Geometry: final body of the model. Coordinates: model frame, mm. A direction names the side the tool comes from. Give positions to 0.01 mm unless a question says otherwise; leave off trailing zeros. Write each loop counter-clockwise with the first axis right and the second up, starting at its lowest first coordinate (ties: lowest second). Pieces come first, ordered by that corner, then holes. Notation, with made-up numbers: (59, -2.5) - (63, -2.5) arc R16 ccw to (63, 12.5) - close; hole circle Ø4 at (-38, 41). An arc over 180 degrees is marked (long way). Use CSV: the item, a comma, the result in double quotes. Start each with the question number.
(1) Line query: probe 1 along X at (y, z) = (244, 98.5); probe 2 along Y at (x, z) = (22.5, 80.5); probe 3 along X at (y, z) = (36, 24.5). Output: solid intervals per line, ascending. Write a range as [from, to].
(2) Section C-C on x = 12. Output: boundary loops of the cut face in (y, z) (3 decimals).
(3) First-contact query: pin 1 Ø1.5 at (x, z) = (184, 43) entering from +Y; pin 2 Ø4 at (y, z) = (277.477, 41.275) entering from +X; pin 3 Ø1.5 at (y, z) = (193.5, 71.5) entering from +X. Flat tips, straight axial feed; report the tip coordinate or a pass-through.
(4) Section B-B on y = 248. Output: boundary loops of the cut face in (x, z) (3 decimals), and give its area (3 significant figures).
(5) Section A-A on z = 89. Output: boundary loops of the cut face in (x, y) (3 decimals).
(6) Reachability of faces 1 (the flat face through (-55.496, 208, 58)), 2 (the flat face through (141.09, -19.38, 57.92)) from +Z, -Z, +X, -X, +Y, -Y: full face, straight path, thin tool, end or side. Return the list, or none.
Autodesk Inventor part; units mm, degrees
ref_plane "YZ Plane" through (0, 0, 0) normal (1, 0, 0) x (0, 1, 0)
ref_plane "XZ Plane" through (0, 0, 0) normal (0, 1, 0) x (-1, 0, 0)
ref_plane "XY Plane" through (0, 0, 0) normal (0, 0, 1) x (1, 0, 0)
sketch "Sketch1" plane through (0, 0, 0) normal (0, 0, 1) x (1, 0, 0)
  line L0 (-58.6709, 290.177) -> (-55.4959, 290.177)
  line L1 (-58.6709, 290.177) -> (-58.6709, 129.0683)
  arc A0 (-58.6709, 129.0683) -> (52.835, -3.8192) centre (76.2666, 129.0683) ccw
  line L2 (52.835, -3.8192) -> (231.8416, -35.3829)
  line L3 (231.8416, -32.1589) -> (231.8416, -35.3829)
  line L4 (231.8416, -32.1589) -> (53.3863, -0.6924)
  arc A1 (-55.4959, 129.0683) -> (53.3863, -0.6924) centre (76.2666, 129.0683) ccw
  line L5 (-55.4959, 129.0683) -> (-55.4959, 290.177)
  point P0 (0, 0)
extrude "Extrusion1" add sketch "Sketch1" along normal blind 117.475
hole "Hole1" at (-55.4959, 277.477, 109.5375) direction (-1, 0, 0) diameter 6.731 depth 25.4 tip angle 118
pattern_linear "Rectangular Pattern1" count 2 spacing 133.35 along (0, -1, 0) of "Hole1"
pattern_linear "Rectangular Pattern2" count 2 spacing 68.2625 along (0, 0, -1) of "Hole1"
hole "Hole2" at (219.3346, -29.9536, 109.5375) direction (-0.1736482, -0.9848078, 0) diameter 6.731 depth 25.4 tip angle 118
pattern_linear "Rectangular Pattern4" count 2 spacing 133.35 along (-0.9848078, 0.1736482, 0) of "Hole2"
properties part number "GE-12070-03"
Check values:
1,probe 1,"x = [-58.67, -55.5]"
1,probe 2,"y = [5.31, 8.77]"
1,probe 3,"x = [-21.44, -17.01]"
2,outline,"(10.418, 0) - (14.042, 0) - (14.042, 117.475) - (10.418, 117.475) - close"
3,pin 1,"stops at y = -23.59"
3,pin 2,"passes through"
3,pin 3,"stops at x = -55.5"
4,outline,"(-58.671, 0) - (-55.496, 0) - (-55.496, 117.475) - (-58.671, 117.475) - close"
4,area,"373 mm²"
5,outline,"(-58.671, 129.068) arc R134.937 ccw to (52.835, -3.819) - (231.842, -35.383) - (231.842, -32.159) - (53.386, -0.692) arc R131.762 cw to (-55.496, 129.068) - (-55.496, 290.177) - (-58.671, 290.177) - close"
6,face 1,"+Z, -Z, +X, +Y"
6,face 2,"+Z, -Z, -X, -Y"
